Build history of the part. All positions in model axes, mm. A direction names the side the tool comes from. Give positions to 0.01 mm unless a question says otherwise; leave off trailing zeros. Order: outer loops, then holes, each group sorted by start corner. A loop starts at its lowest first (then second) coordinate and runs counter-clockwise, first axis right, second up. Notation, with made-up numbers: (77.25, 16) - (117.25, 16) arc R15 cw to (117.25, 37) - close; hole circle Ø6 at (24, 89.5). An arc over 180 degrees is marked (long way). Use a Markdown table: item, result. Add a question column.
(1) Wall check: line 1 (X direction, y = -6, z = -12.25); line 2 (Z direction, x = -11, y = -2.5). Give the ranges that are in metal, low to high.
(2) Slice it at C-C (z = -12.5). Write the cut outline in (x, y), then the cut area to 3 significant figures.
(3) Slice it at A-A (y = -3.75). Write the cut outline in (x, z).
(4) Which spindle directions (+Z, -Z, +X, -X, +Y, -Y) get a long thin tool onto all of the face, cutting with end or side? Do faces 1 (the face through (0, -10, -7)), 2 (the face through (29, 0, -2)). Say none if no direction does.
(5) Flat gauge pins, fed straight in: pin 1 (4.5 mm diameter, centred on y = -7, z = -9, fed in from -X); pin 2 (6 mm diameter, centred on x = 7, z = 1.5, fed in from +Y); pin 3 (5 mm diameter, centred on x = -18.5, y = -3, fed in from -Z). Where does each tip first touch, or does it go through?
(6) Slice it at B-B (x = -9.5). Write the cut outline in (y, z).
from build123d import *

# Parameters (mm, degrees)
PAD_DEPTH = 20


with BuildPart() as part:
    # Sketch → Pad (new body)
    with BuildSketch(Plane.XZ):
        Polygon((-40, 10), (-40, 0), (0, 0), (0, -15), (75, -15), (75, 10), align=None)
    extrude(amount=PAD_DEPTH)


solid = part.part
Solution:
| question | item | result |
|---|---|---|
| 1 | line 1 | 0 to 75 |
| 1 | line 2 | 0 to 10 |
| 2 | outline | (0, -20) - (75, -20) - (75, 0) - (0, 0) - close |
| 2 | area | 1,500 mm2 |
| 3 | outline | (-40, 0) - (0, 0) - (0, -15) - (75, -15) - (75, 10) - (-40, 10) - close |
| 4 | face 1 | -Z, -X, +Y, -Y |
| 4 | face 2 | +Z, -Z, +X, -X, +Y |
| 5 | pin 1 | x = 0 |
| 5 | pin 2 | y = 0 |
| 5 | pin 3 | z = 0 |
| 6 | outline | (-20, 0) - (0, 0) - (0, 10) - (-20, 10) - close |
